from build123d import *

# Parameters (mm, degrees)
PAD050_DEPTH            = 57
POCKET044_DEPTH         = 16
POCKET046_DEPTH         = 16
SKETCH090_W             = 20
SKETCH090_H             = 25
POCKET045_DEPTH         = 10
BODY022_PLACEMENT_ANGLE = 180


with BuildPart() as part:
    # Sketch092 → Pad050 (new body)
    with BuildSketch(Plane.YZ):
        Polygon((54.734671, -10), (98.357923, 72.85), (87.056432, 72.85), (43.43318, -10), align=None)
    extrude(amount=-PAD050_DEPTH)

    # Sketch089 (on Face5 of Pad050) → Pocket044 (cut)
    with BuildSketch(Plane.YZ):
        Polygon((43.43318, -10), (54.734671, -10), (60, 0), (48.698509, 0), align=None)
    extrude(amount=-POCKET044_DEPTH, mode=Mode.SUBTRACT)

    # Sketch094 (on Face6 of Pocket044) → Pocket046 (cut)
    with BuildSketch(Plane(origin=(-57, 0, 0), x_dir=(0, 1, 0), z_dir=(-1, 0, 0))):
        Polygon((43.43318, 10), (54.734671, 10), (60, 0), (48.698509, 0), align=None)
    extrude(amount=-POCKET046_DEPTH, mode=Mode.SUBTRACT)

    # Sketch090 (on Face5 of Pocket046) → Pocket045 (cut)
    with BuildSketch(Plane(origin=(0, 0, 72.85), x_dir=(0, -1, 0), z_dir=(0, 0, 1))):
        with Locations((-88.357923, -28.5)):
            Rectangle(SKETCH090_W, SKETCH090_H)
    extrude(amount=-POCKET045_DEPTH, mode=Mode.SUBTRACT)


with BuildPart() as part_1:
    # Body022 placement: moved
    add(part.part.moved(Location((-57, 295, 0))).rotate(Axis((-57, 295, 0), (0, 0, 1)), BODY022_PLACEMENT_ANGLE))


solid = part_1.part
Work out the finished part from the listing and answer in its coordinate system (mm). A direction names the side the tool comes from. Coordinates: 2 decimals unless noted, no trailing zeros. Order: outer loops, then holes, each group sorted by start corner. A loop starts at its lowest first (then second) coordinate and runs counter-clockwise, first axis right, second up. Notation, with made-up numbers: (-3.75, 62) - (53.25, 62) arc R18 ccw to (53.25, 78) - close; hole circle Ø1 at (84, -6). An arc over 180 degrees is marked (long way). Put each result on its own line as item: value. Start each with the question number.
1) Find the intervals of material crossed by line 1 (Y direction, x = -50.5, z = 25); line 2 (Y direction, x = -2.5, z = 55.5); line 3 (Z direction, x = -12, y = 220.5), in increasing order. Write a range as from..to.
2) Find section A-A (y = 238). Give the vertices of the cut face in (x, z).
3) For a pull along X with two mould halves and no side action, classify faces 6 (the flat face through (-16, 243, -5)), 7 (the flat face through (-16, 205, 68)), 8 (the flat face through (-57, 222, 37)), 9 (the flat face through (-49, 241, 0)) as released by +X, released by -X, zero draft, split by the parting line, or undercut.
4) Find section D-D (y = 204). Give the vertices of the cut face in (x, z), plus the area to 3 significant figures.
5) Find section C-C (x = -37). Give the vertices of the cut face in (y, z).
6) For faces 1 (the flat face through (-41, 205, 68)), 2 (the flat face through (-41, 243, -5)), 3 (the flat face through (-8, 241, 0)), 4 (the flat face through (-28.899, 218.759, 30.845)), 5 (the flat face through (-49, 202, 72.85)), determine the directions among +Z, -Z, +X, -X, +Y, -Y from which every point of the face is accessible in a straight line to the end or side of a thin tool.
7) Find section B-B (z = 66). Give the vertices of the cut face in (x, y).
8) Flat-ended cylindrical pins translate along their axes: pin 1 (3 mm diameter, centred on x = -41, y = 243, fed in from +Z); pin 2 (2 mm diameter, centred on x = -40, z = 49.5, fed in from -Y); pin 3 (5.5 mm diameter, centred on x = -28.5, y = 206.5, fed in from +Z); pin 4 (10 mm diameter, centred on y = 205, z = 49.5, fed in from -X). Find the tip coordinate at first contact, or state that the pin passes through.
Results list:
1. line 1: y = 221.84..233.14
1. line 2: y = 205.78..217.08
1. line 3: z = 27.54..49
2. outline: (-57, 0) - (-41, 0) - (-41, -5.7) - (-16, -5.7) - (-16, 0) - (0, 0) - (0, 15.77) - (-57, 15.77) - close
3. face 6: released by +X
3. face 7: undercut
3. face 8: released by -X
3. face 9: zero draft
4. outline: (-57, 58.88) - (0, 58.88) - (0, 72.85) - (-16, 72.85) - (-16, 62.85) - (-41, 62.85) - (-41, 72.85) - (-57, 72.85) - close
4. area: 547 mm^2
5. outline: (201.91, 62.85) - (240.27, -10) - (251.57, -10) - (213.21, 62.85) - close
6. face 1: +Z, +Y, -Y
6. face 2: -Z, -X, +Y, -Y
6. face 3: -Z, +X, +Y, -Y
6. face 4: -Z, +X, -X, -Y
6. face 5: +Z, +X, -X, +Y, -Y
7. outline: (-57, 200.25) - (-41, 200.25) - (-41, 211.55) - (-57, 211.55) - close; (-16, 200.25) - (0, 200.25) - (0, 211.55) - (-16, 211.55) - close
8. pin 1: stops at z = 9.12
8. pin 2: stops at y = 208.41
8. pin 3: stops at z = 62.85
8. pin 4: stops at x = -57
